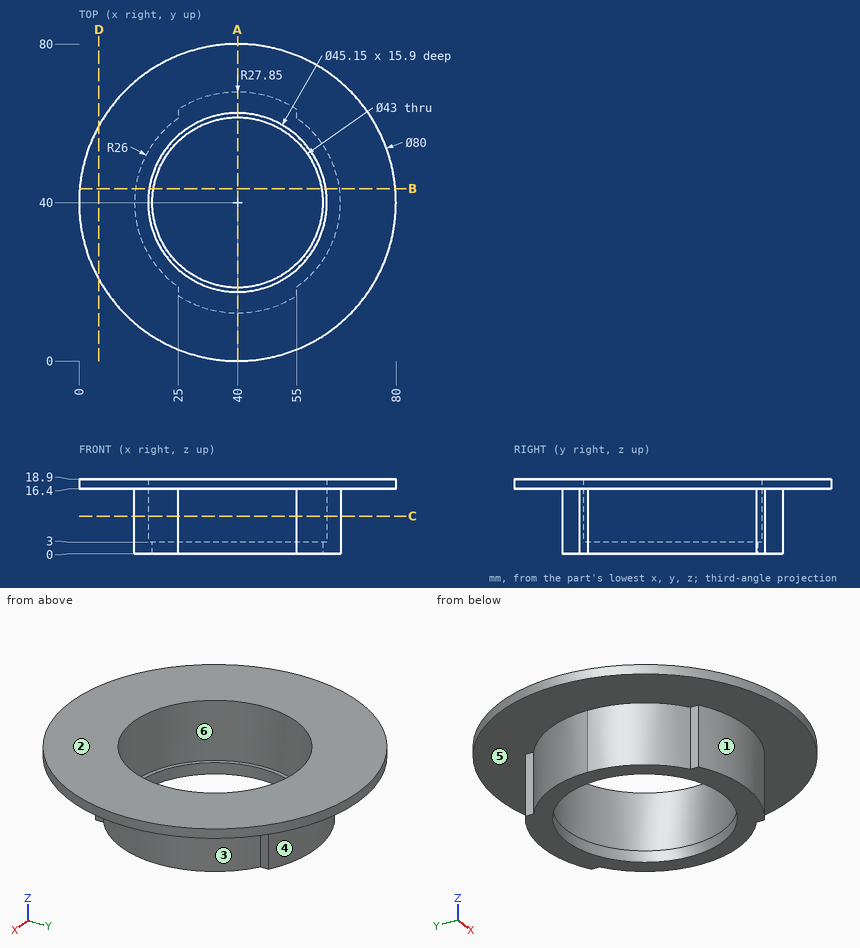
The figure shows three views and two pictorial views of one solid part (mm, origin at its lowest corner). Answer the questions. A direction names the side the tool comes from. Give positions to 0.01 mm unless a question says otherwise; leave off trailing zeros. Loops run counter-clockwise (first coordinate to the right, second up) from the corner with the lowest first, then second, coordinate; pieces in that order, holes last. Notation, with made-up numbers: (59, 88) -> (81, 88) arc R22 cw to (81, 117) -> close; hole circle Ø4 at (35.5, 61). An arc over 180 degrees is marked (long way). Use a Markdown table: item, result. Add a question column.
1. Find the intervals of material crossed by probe 1 along Y at (x, z) = (40, 1.3); probe 2 along Z at (x, y) = (76, 26.5); probe 3 along X at (y, z) = (49, 17), in increasing order.
2. Section A-A on x = 40 is taken. Determine the outline of the cut face in (y, z) (3 decimals), and give its area (3 significant figures).
3. Flat-ended cylindrical pins translate along their axes: pin 1 Ø1 at (x, z) = (27.5, 2) entering from -Y; pin 2 Ø24 at (x, y) = (37, 47) entering from -Z; pin 3 Ø1.5 at (y, z) = (66, 12) entering from +X; pin 4 Ø0.7 at (y, z) = (17, 8) entering from -X. Find the tip coordinate at first contact, or state that the pin passes through.
4. Determine the mould class of the marked faces 3, 4, 5 and 6 for opening direction X: released by +X, released by -X, zero draft, split by the parting line, or undercut.
5. Section C-C on z = 9.5 is taken. Determine the outline of the cut face in (x, y) (3 decimals), and give its area (3 significant figures).
6. Section D-D on x = 5 is taken. Determine the outline of the cut face in (y, z), and give its area (3 significant figures).
7. For the marked faces 1 and 2, determine the directions among +Z, -Z, +X, -X, +Y, -Y from which every point of the face is accessible in a straight line to the end or side of a thin tool.
8. Section B-B on y = 43.5 is taken. Determine the outline of the cut face in (x, z), and give its area (3 significant figures).
Results below:
| question | item | result |
|---|---|---|
| 1 | probe 1 | y = 12.15 to 18.5, 61.5 to 67.85 |
| 1 | probe 2 | z = 16.4 to 18.9 |
| 1 | probe 3 | x = 1.03 to 19.3, 60.7 to 78.97 |
| 2 | outline | (0, 16.4) -> (12.15, 16.4) -> (12.15, 0) -> (18.5, 0) -> (18.5, 3) -> (17.425, 3) -> (17.425, 18.9) -> (0, 18.9) -> close; (61.5, 0) -> (67.85, 0) -> (67.85, 16.4) -> (80, 16.4) -> (80, 18.9) -> (62.575, 18.9) -> (62.575, 3) -> (61.5, 3) -> close |
| 2 | area | 267 mm^2 |
| 3 | pin 1 | stops at y = 14.87 |
| 3 | pin 2 | passes through |
| 3 | pin 3 | stops at x = 51.75 |
| 3 | pin 4 | stops at x = 25 |
| 4 | face 3 | released by +X |
| 4 | face 4 | split by the parting line |
| 4 | face 5 | zero draft |
| 4 | face 6 | undercut |
| 5 | outline | (25, 16.535) arc R27.85 ccw to (55, 16.535) -> (55, 18.763) arc R26 ccw to (55, 61.237) -> (55, 63.465) arc R27.85 ccw to (25, 63.465) -> (25, 61.237) arc R26 ccw to (25, 18.763) -> close; hole circle Ø45.15 at (40, 40) |
| 5 | area | 640 mm^2 |
| 6 | outline | (20.64, 16.4) -> (59.36, 16.4) -> (59.36, 18.9) -> (20.64, 18.9) -> close |
| 6 | area | 96.8 mm^2 |
| 7 | face 1 | -Z, -Y |
| 7 | face 2 | +Z, +X, -X, +Y, -Y |
| 8 | outline | (0.15, 16.4) -> (14.24, 16.4) -> (14.24, 0) -> (18.79, 0) -> (18.79, 3) -> (17.7, 3) -> (17.7, 18.9) -> (0.15, 18.9) -> close; (61.21, 0) -> (65.76, 0) -> (65.76, 16.4) -> (79.85, 16.4) -> (79.85, 18.9) -> (62.3, 18.9) -> (62.3, 3) -> (61.21, 3) -> close |
| 8 | area | 208 mm^2 |
